Design review of the part built by this model. Coordinates are the model's own, in mm. A direction names the side the tool comes from. Give positions to 0.01 mm unless a question says otherwise; leave off trailing zeros. Write each loop counter-clockwise with the first axis right and the second up, starting at its lowest first coordinate (ties: lowest second). Pieces come first, ordered by that corner, then holes. Notation, with made-up numbers: (85, -39.75) - (96, -39.75) arc R17 ccw to (96, -14.75) - close; hole circle Ø11 at (-10, 65). An arc over 180 degrees is marked (long way). Use a Markdown table: item, result. Add a question column.
```python
from build123d import *

# Parameters (mm, degrees)
BOSS_EXTRUDE1_DEPTH = 8
SKETCH2_R           = 2.4
BOSS_EXTRUDE2_DEPTH = 1.6
SHELL1_T            = -1.6


with BuildPart() as part:
    # Sketch1 → Boss-Extrude1 (new body)
    with BuildSketch(Plane(origin=(0, 0, 0), x_dir=(0, 0, -1), z_dir=(1, 0, 0))):
        Polygon((0, 0), (24, 0), (24, 1.6), (8, 9.6), (0, 9.6), align=None)
    extrude(amount=BOSS_EXTRUDE1_DEPTH)

    # Sketch2 → Boss-Extrude2 (add)
    with BuildSketch(Plane(origin=(0, 9.6, 0), x_dir=(1, 0, 0), z_dir=(0, 1, 0))):
        with Locations(Location((4, 4, 0), (0, 0, 270))):
            Circle(SKETCH2_R)
    extrude(amount=BOSS_EXTRUDE2_DEPTH)

    # Shell1
    shell1_openings = [part.faces().sort_by_distance(p)[0] for p in [
        (4, 0, -12),
    ]]
    offset(amount=SHELL1_T, openings=shell1_openings, kind=Kind.INTERSECTION)


solid = part.part
```
(1) Mouldability with a two-part tool opening along X and no side actions: class faces 1 (the face through (6.024, 10.389, -2.71)), 2 (the face through (4, 11.2, -4)), 3 (the face through (3, 8, -5)) as +X half, -X half, draft (parallel to the pull), parting line (faces both ways), or undercut.
(2) Add section B-B (y = 5). State the section outline as (x, z) points.
(3) Add section A-A (x = 4). State the section outline as (y, z) points.
(4) Tool access review of faces 4 (the face through (7, 0, -12)), 5 (the face through (6, 9.6, -2)), 6 (the face through (4, 9.6, -4)): name each direction out of +Z, -Z, +X, -X, +Y, -Y from which nothing blocks a thin tool from reaching the whole face with its end or side.
(5) Add section C-C (z = -4). State the section outline as (x, y) points, and give its area (3 significant figures).
(6) For line 1 along X through (y, z) = (3.5, -11.75); line 2 along X through (y, z) = (8.4, -4); line 3 along Z through (x, y) = (4, 9.1), list the stretches that pass through material, from the lowest coordinate up.
(7) Insertion check: pin 1 (1 mm diameter, centred on x = 4, y = 6, fed in from -Z); pin 2 (1 mm diameter, centred on x = 4, z = -4, fed in from -Y); pin 3 (1.3 mm diameter, centred on x = 4, z = -3.5, fed in from -Y); pin 4 (4 mm diameter, centred on x = 3, z = -3.5, fed in from -Y). Each pin has a flat end and moves straight along its axis. Give the tip position at first contact, or say it passes through.
(8) Add section D-D (x = 1.25). State the section outline as (y, z) points, and give its area (3 significant figures).
Answers follow:
| question | item | result |
|---|---|---|
| 1 | face 1 | parting line |
| 1 | face 2 | draft |
| 1 | face 3 | undercut |
| 2 | outline | (0, -17.2) - (8, -17.2) - (8, 0) - (0, 0) - close; hole (1.6, -13.62) - (6.4, -13.62) - (6.4, -1.6) - (1.6, -1.6) - close |
| 3 | outline | (0, -24) - (1.6, -24) - (9.6, -8) - (9.6, -6.4) - (11.2, -6.4) - (11.2, -1.6) - (9.6, -1.6) - (9.6, 0) - (0, 0) - (0, -1.6) - (8, -1.6) - (8, -3.2) - (9.6, -3.2) - (9.6, -4.8) - (8, -4.8) - (8, -7.62) - (0.61, -22.4) - (0, -22.4) - close |
| 4 | face 4 | +Z, -Z, +X, -X, -Y |
| 4 | face 5 | +Y |
| 4 | face 6 | -Y |
| 5 | outline | (0, 0) - (1.6, 0) - (1.6, 8) - (3.2, 8) - (3.2, 9.6) - (4.8, 9.6) - (4.8, 8) - (6.4, 8) - (6.4, 0) - (8, 0) - (8, 9.6) - (6.4, 9.6) - (6.4, 11.2) - (1.6, 11.2) - (1.6, 9.6) - (0, 9.6) - close |
| 5 | area | 43.5 mm^2 |
| 6 | line 1 | 0 to 1.6, 6.4 to 8 |
| 6 | line 2 | 0 to 3.2, 4.8 to 8 |
| 6 | line 3 | -9 to -4.8, -3.2 to 0 |
| 7 | pin 1 | z = -16.2 |
| 7 | pin 2 | y = 9.6 |
| 7 | pin 3 | y = 8 |
| 7 | pin 4 | y = 0 |
| 8 | outline | (0, -24) - (1.6, -24) - (9.6, -8) - (9.6, 0) - (0, 0) - close |
| 8 | area | 166 mm^2 |
